Autodesk Inventor part; units mm, degrees
ref_plane "Plano de trabajo3" through (0, 30, 31) normal (0, 0, 1) x (1, 0, 0)
ref_plane "Plano de trabajo4" through (68.3847, 0, 31) normal (1, 0, 0) x (0, 1, 0)
ref_plane "Plano de trabajo5" through (11, 0, 31) normal (0, 0, 1) x (1, 0, 0)
sketch "Boceto1" plane through (0, 0, 0) normal (0, 1, 0) x (-1, 0, 0)
  line L0 (0, 0) -> (-22, 0)
  line L1 (-22, 0) -> (-22, 62)
  line L2 (-22, 62) -> (0, 62)
  line L3 (0, 62) -> (0, 0)
  dimension "d0" = 62
  dimension "d1" = 22
extrude "Extrusión1" add sketch "Boceto1" along normal blind 30
sketch "Boceto2" plane through (22, 0, 62) normal (1, 0, 0) x (0, 0, -1)
  line L0 (62, 0) -> (0, 0)
  line L1 (62, 0) -> (62, 30)
  line L2 (0, 30) -> (62, 30)
  line L3 (0, 0) -> (0, 30)
  line L4 (2, 28) -> (60, 28)
  line L5 (60, 28) -> (60, 2)
  line L6 (60, 2) -> (2, 2)
  line L7 (2, 2) -> (2, 28)
  dimension "d4" = 2
  dimension "d5" = 2
  dimension "d6" = 2
  dimension "d7" = 2
extrude "Extrusión2" cut sketch "Boceto2" against normal blind 30 contours L4 L5 L6 L7
sketch "Boceto3" plane through (0, 0, 0) normal (0, -1, 0) x (1, 0, 0)
  line L0 (0, 0) -> (22, 0)
  line L1 (22, 62) -> (0, 62)
  line L2 (22, 62) -> (7, 62)
  line L3 (7, 62) -> (7, 31)
  circle A0 centre (7, 31) radius 1
  dimension "d10" = 15
  dimension "d11" = 31
  dimension "d12" = 2
extrude "Extrusión3" cut sketch "Boceto3" against normal blind 15
sketch "Boceto4" plane through (0, 0, 62) normal (0, 0, 1) x (1, 0, 0)
  line L0 (22, 0) -> (0, 0)
  line L1 (22, 0) -> (22, 30)
  line L2 (0, 30) -> (22, 30)
  line L3 (0, 0) -> (0, 30)
sketch "Boceto5" plane through (0, 0, 62) normal (0, 0, 1) x (1, 0, 0)
  line L0 (22, 0) -> (0, 0)
  line L1 (22, 0) -> (22, 30)
  line L2 (0, 30) -> (22, 30)
  line L3 (0, 0) -> (0, 30)
sketch "Boceto7" plane through (0, 0, 62) normal (0, 0, 1) x (1, 0, 0)
  line L0 (22, 0) -> (0, 0)
  line L1 (22, 0) -> (22, 30)
  line L2 (0, 30) -> (22, 30)
  line L3 (0, 0) -> (0, 30)
  line L4 (0, 30) -> (22, 30)
  line L5 (22, 30) -> (22, 0)
  line L6 (22, 0) -> (0, 0)
  line L7 (0, 0) -> (0, 30)
  line L8 (22, 0) -> (11, 0)
  line L9 (11, 0) -> (11, 15)
  line L10 (11, 15) -> (22, 15)
  line L11 (22, 15) -> (22, 0)
  dimension "d17" = 15
  dimension "d18" = 11
sketch "Boceto9" plane through (0, 0, 62) normal (0, 0, 1) x (1, 0, 0)
  line L0 (22, 0) -> (0, 0)
  line L1 (22, 0) -> (22, 30)
  line L2 (0, 30) -> (22, 30)
  line L3 (0, 0) -> (0, 30)
sketch "Boceto10" plane through (22, 0, 62) normal (1, 0, 0) x (0, 0, -1)
  line L0 (62, 0) -> (0, 0)
  line L1 (0, 30) -> (62, 30)
  line L2 (0, 30) -> (31, 30) construction
  line L3 (31, 30) -> (31, 0) construction
  line L4 (0, 0) -> (-20, 0)
  line L5 (-20, 0) -> (-20, 15)
  line L6 (-20, 15) -> (0, 15)
  line L7 (0, 15) -> (0, 0)
  line L8 (62, 0) -> (62, 30)
  line L9 (62, 0) -> (82, 0)
  line L10 (82, 0) -> (82, 15)
  line L11 (82, 15) -> (62, 15)
  line L12 (0, 30) -> (62, 30)
  line L13 (62, 30) -> (62, 0)
  line L14 (62, 0) -> (0, 0)
  line L15 (0, 0) -> (0, 30)
  line L16 (2, 28) -> (60, 28)
  line L17 (60, 28) -> (60, 2)
  line L18 (60, 2) -> (2, 2)
  line L19 (2, 2) -> (2, 28)
  dimension "d20" = 31
  dimension "d21" = 20
  dimension "d22" = 15
extrude "Extrusión4" add sketch "Boceto10" against normal blind 11 contours L4 L5 L6 L7
ref_plane "Plano de trabajo3" through (0, 30, 31) normal (0, 0, 1) x (1, 0, 0)
mirror "Simetría1" about plane through (0, 30, 31) normal (0, 0, 1) of "Extrusión4"
sketch "Boceto11" plane through (0, 0, 0) normal (0, -1, 0) x (1, 0, 0)
  line L0 (11, 0) -> (11, -20)
  line L1 (0, 62) -> (0, 0)
  line L2 (11, 82) -> (33, 82)
  line L3 (33, 82) -> (33, 84)
  line L4 (33, 84) -> (11, 84)
  line L5 (11, 84) -> (11, 82)
  line L6 (0, 31) -> (103.8517, 31) construction
  line L7 (11, 62) -> (11, 0) construction
  circle A0 centre (11, 31) radius 57.3847 construction
  line L8 (33, 84) -> (51.3255, 71.8272)
  line L9 (51.3255, 71.8272) -> (68.3847, 31)
  line L10 (33, 82) -> (50.3824, 70.4536)
  line L11 (50.3824, 70.4536) -> (66.8677, 31)
  line L12 (68.3847, 31) -> (66.8677, 31)
  line L13 (11, -20) -> (33, -20)
  line L14 (33, -20) -> (33, -22)
  line L15 (33, -22) -> (11, -22)
  line L16 (11, -22) -> (11, -20)
  line L17 (33, -22) -> (51.3255, -9.8272)
  line L18 (51.3255, -9.8272) -> (68.3847, 31)
  line L19 (33, -20) -> (50.3824, -8.4536)
  line L20 (50.3824, -8.4536) -> (66.8677, 31)
  dimension "d25" = 22
  dimension "d26" = 2
  dimension "d27" = 22
  dimension "d28" = 39.4536
extrude "Extrusión5" add sketch "Boceto11" against normal blind 100
ref_plane "Plano de trabajo4" through (68.3847, 0, 31) normal (1, 0, 0) x (0, 1, 0)
sketch "Boceto12" plane through (68.3847, 0, 31) normal (1, 0, 0) x (0, 1, 0)
  point P0 (0, -31)
sketch "Boceto13" plane through (68.3847, 0, 31) normal (1, 0, 0) x (0, 1, 0)
  line L0 (0, 40.8272) -> (0, 53)
  line L1 (0, 40.8272) -> (100, 40.8272)
  line L2 (100, 53) -> (100, 40.8272)
  line L3 (0, 53) -> (100, 53)
  line L4 (0, 0) -> (0, 40.8272)
  line L5 (0, 0) -> (100, 0)
  line L6 (100, 40.8272) -> (100, 0)
  line L7 (0, 40.8272) -> (100, 40.8272)
  line L8 (0, -40.8272) -> (0, 0)
  line L9 (0, -40.8272) -> (100, -40.8272)
  line L10 (100, 0) -> (100, -40.8272)
  line L11 (0, 0) -> (100, 0)
  line L12 (0, -53) -> (0, -40.8272)
  line L13 (0, -53) -> (100, -53)
  line L14 (100, -40.8272) -> (100, -53)
  line L15 (0, -40.8272) -> (100, -40.8272)
  line L16 (0, 0) -> (20, 0) construction
  line L17 (0, -51) -> (100, -51)
  line L18 (20, 0) -> (32.1544, -40.8272)
  line L19 (32.1544, -40.8272) -> (53.0672, -51)
  line L20 (32.1544, -40.8272) -> (42.1544, -40.8272) construction
  line L21 (20, 0) -> (40, 0) construction
  line L22 (40, 0) -> (42.1544, -40.8272)
  line L23 (42.1544, -40.8272) -> (53.0672, -51)
  line L24 (40, 0) -> (20, 0)
  line L25 (20, 0) -> (0, 0)
  line L26 (42.1544, -40.8272) -> (32.1544, -40.8272)
  line L27 (0, 51) -> (100, 51)
  line L28 (20, 0) -> (32.1544, 40.8272)
  line L29 (32.1544, 40.8272) -> (53.0672, 51)
  line L30 (40, 0) -> (42.1544, 40.8272)
  line L31 (42.1544, 40.8272) -> (53.0672, 51)
  point P0 (0, -31)
  dimension "d32" = 20
  dimension "d33" = 10
  dimension "d34" = 20
  dimension "d35" = 20.9128
extrude "Extrusión6" cut sketch "Boceto13" against normal blind 40 contours L5 L22 L9 L18 | L9 L23 L19
ref_plane "Plano de trabajo5" through (11, 0, 31) normal (0, 0, 1) x (1, 0, 0)
mirror "Simetría2" about plane through (11, 0, 31) normal (0, 0, 1) of "Extrusión6"
sketch "Boceto14" plane through (68.3847, 0, 31) normal (1, 0, 0) x (0, 1, 0)
  line L0 (32.1544, 40.8272) -> (53.0672, 51)
  line L1 (53.0672, 51) -> (42.1544, 40.8272)
  line L2 (42.1544, 40.8272) -> (100, 40.8272)
  line L3 (100, 53) -> (100, 40.8272)
  line L4 (0, 53) -> (100, 53)
  line L5 (0, 40.8272) -> (0, 53)
  line L6 (0, 40.8272) -> (32.1544, 40.8272)
  line L7 (42.1544, 40.8272) -> (40, 0)
  line L8 (40, 0) -> (100, 0)
  line L9 (100, 40.8272) -> (100, 0)
  line L10 (42.1544, 40.8272) -> (100, 40.8272)
  line L11 (40, 0) -> (42.1544, -40.8272)
  line L12 (42.1544, -40.8272) -> (100, -40.8272)
  line L13 (100, 0) -> (100, -40.8272)
  line L14 (40, 0) -> (100, 0)
  line L15 (53.0672, -51) -> (32.1544, -40.8272)
  line L16 (0, -40.8272) -> (32.1544, -40.8272)
  line L17 (0, -53) -> (0, -40.8272)
  line L18 (0, -53) -> (100, -53)
  line L19 (100, -40.8272) -> (100, -53)
  line L20 (42.1544, -40.8272) -> (100, -40.8272)
  line L21 (42.1544, -40.8272) -> (53.0672, -51)
  line L22 (32.1544, -40.8272) -> (20, 0)
  line L23 (0, 0) -> (20, 0)
  line L24 (0, -40.8272) -> (0, 0)
  line L25 (0, -40.8272) -> (32.1544, -40.8272)
  line L26 (20, 0) -> (32.1544, 40.8272)
  line L27 (0, 40.8272) -> (32.1544, 40.8272)
  line L28 (0, 0) -> (0, 40.8272)
  line L29 (0, 0) -> (20, 0)
  line L30 (100, 53) -> (80, 53)
  line L31 (80, 53) -> (80, -53)
  line L32 (100, -53) -> (100, 53)
  line L33 (80, -53) -> (100, -53)
  point P0 (0, -31)
  dimension "d38" = 20
extrude "Extrusión7" cut sketch "Boceto14" against normal blind 40 contours L31 L4 L3 L2 | L2 L9 L8 L31 | L8 L13 L12 L31 | L12 L19 L18 L31
sketch "Boceto15" plane through (0, 30, 0) normal (0, 1, 0) x (1, 0, 0)
  line L0 (0, 0) -> (0, -62)
  line L1 (22, -62) -> (22, 0)
  line L2 (0, -31) -> (22, -31) construction
  line L3 (22, -31) -> (22, -19.5) construction
  line L4 (22, -31) -> (22, -42.5) construction
  line L5 (0, -19.5) -> (55, -19.5)
  line L6 (55, -19.5) -> (55, -14.5)
  line L7 (55, -14.5) -> (22, -14.5)
  line L8 (22, -14.5) -> (22, -9.5)
  line L9 (22, -9.5) -> (0, -9.5)
  line L10 (0, -19.5) -> (0, -9.5)
  line L11 (0, -9.5) -> (0, -19.5)
  line L12 (0, -42.5) -> (55, -42.5)
  line L13 (55, -42.5) -> (55, -47.5)
  line L14 (55, -47.5) -> (22, -47.5)
  line L15 (22, -47.5) -> (22, -52.5)
  line L16 (22, -52.5) -> (0, -52.5)
  line L17 (0, -52.5) -> (0, -42.5)
  dimension "d41" = 11.5
  dimension "d42" = 11.5
  dimension "d43" = 55
  dimension "d44" = 5
  dimension "d45" = 5
extrude "Extrusión8" add sketch "Boceto15" along normal blind 25 contours L9 L1 L5 L0 | L12 L1 L16 L0 | L1 L7 L6 L5 | L12 L13 L14 L1
ref_plane "Plano de trabajo6" through (55, 42.5, 47.5) normal (1, 0, 0) x (0, 0, -1)
sketch "Boceto16" plane through (55, 42.5, 47.5) normal (1, 0, 0) x (0, 0, -1)
  line L0 (28, -12.5) -> (33, -12.5)
  line L1 (33, -12.5) -> (33, 12.5)
  line L2 (28, 12.5) -> (33, 12.5)
  line L3 (28, -12.5) -> (28, 12.5)
  line L4 (0, -12.5) -> (5, -12.5)
  line L5 (5, -12.5) -> (5, 12.5)
  line L6 (0, 12.5) -> (5, 12.5)
  line L7 (0, -12.5) -> (0, 12.5)
  line L8 (0, -12.5) -> (10, -12.5)
  line L9 (10, -12.5) -> (10, 12.5)
  line L10 (10, 12.5) -> (0, 12.5)
  line L11 (0, 12.5) -> (0, -12.5)
  line L12 (5, 0) -> (16.5, 0) construction
  line L13 (-12.5, -40.5) -> (-12.5, -14.5) construction
  line L14 (-12.5, -14.5) -> (45.5, -14.5) construction
  line L15 (45.5, -14.5) -> (45.5, -40.5) construction
  line L16 (45.5, -40.5) -> (-12.5, -40.5) construction
  line L17 (67.5, -42.5) -> (-34.5, -42.5) construction
  line L18 (67.5, -27.5) -> (67.5, -42.5) construction
  line L19 (47.5, -27.5) -> (67.5, -27.5) construction
  line L20 (47.5, -27.5) -> (47.5, -12.5) construction
  line L21 (38, -12.5) -> (47.5, -12.5) construction
  line L22 (38, -12.5) -> (38, 12.5) construction
  line L23 (33, 12.5) -> (38, 12.5) construction
  line L24 (33, -12.5) -> (33, 12.5) construction
  line L25 (28, -12.5) -> (33, -12.5) construction
  line L26 (5, -12.5) -> (28, -12.5) construction
  line L27 (0, -12.5) -> (5, -12.5) construction
  line L28 (0, -12.5) -> (0, 12.5) construction
  line L29 (-5, 12.5) -> (0, 12.5) construction
  line L30 (-5, -12.5) -> (-5, 12.5) construction
  line L31 (-14.5, -12.5) -> (-5, -12.5) construction
  line L32 (-14.5, -27.5) -> (-14.5, -12.5) construction
  line L33 (-14.5, -27.5) -> (-34.5, -27.5) construction
  line L34 (-34.5, -27.5) -> (-34.5, -42.5) construction
  line L35 (16.5, -12.5) -> (16.5, -3.1507) construction
  line L36 (33, -12.5) -> (28, -12.5)
  line L37 (33, 12.5) -> (28, 12.5)
  line L38 (33, -12.5) -> (33, 12.5)
  line L39 (33, -12.5) -> (23, -12.5)
  line L40 (23, -12.5) -> (23, 12.5)
  line L41 (23, 12.5) -> (33, 12.5)
  point P0 (47.5, -42.5)
  dimension "d49" = 25
  dimension "d50" = 11.5
  dimension "d51" = 11.5
extrude "Extrusión9" add sketch "Boceto16" along normal blind 2 contours L7 L6 L5 L4 | L5 L10 L9 L8
ref_plane "Plano de trabajo7" through (33, 0, 31) normal (0, 0, -1) x (-1, 0, 0)
mirror "Simetría3" about plane through (33, 0, 31) normal (0, 0, -1) of "Extrusión9"
ref_plane "Plano de trabajo8" through (55, 42.5, 24.5) normal (-1, 0, 0) x (0, 0, 1)
sketch "Boceto17" plane through (55, 42.5, 24.5) normal (-1, 0, 0) x (0, 0, 1)
  line L0 (-5, -12.5) -> (-5, 12.5)
  line L1 (-5, -12.5) -> (0, -12.5)
  line L2 (0, -12.5) -> (0, 12.5)
  line L3 (0, 12.5) -> (-5, 12.5)
  line L4 (18, -12.5) -> (18, 12.5)
  line L5 (13, 12.5) -> (18, 12.5)
  line L6 (13, -12.5) -> (13, 12.5)
  line L7 (18, -12.5) -> (13, -12.5)
  line L8 (18, -12.5) -> (18, -5.5) construction
  line L9 (18, -5.5) -> (15.5, -5.5) construction
  circle A0 centre (15.5, -5.5) radius 1.5 construction
  circle A1 centre (15.5, -5.5) radius 1.5
  circle A2 centre (15.5, 6.5997) radius 1.5
  circle A3 centre (-2.5, 6.5997) radius 1.5
  circle A4 centre (-2.5, -5.5) radius 1.5
  point P0 (-24.5, -42.5)
  dimension "d54" = 7
  dimension "d55" = 2.5
  dimension "d56" = 3
  dimension "d57" = 3
  dimension "d58" = 3
  dimension "d59" = 3
  dimension "d60" = 3
extrude "Extrusión10" cut sketch "Boceto17" against normal blind 5 contours A1 | A2 | A3 | A4
sketch "Boceto18" plane through (0, 0, 0) normal (0, -1, 0) x (1, 0, 0)
  line L0 (0, 62) -> (-88, 62)
  line L1 (-88, 62) -> (-88, 53.488)
  line L2 (-88, 53.488) -> (0, 53.488)
  line L3 (0, 53.488) -> (0, 62)
  dimension "d63" = 88
extrude "Extrusión11" add sketch "Boceto18" against normal blind 2
mirror "Simetría4" about plane through (33, 0, 31) normal (0, 0, -1) of "Extrusión11"
fillet "Empalme1" radius 2 1 edges at (27.5, 55, 19.5)
fillet "Empalme2" radius 2 1 edges at (27.5, 55, 42.5)
fillet "Empalme3" radius 2 1 edges at (56, 55, 37.5)
fillet "Empalme4" radius 2 1 edges at (56, 55, 24.5)
fillet "Empalme5" radius 2 1 edges at (11, 15, 72)
fillet "Empalme6" radius 2 1 edges at (11, 15, -10)
fillet "Empalme7" radius 2 1 edges at (22, 15, 72)
fillet "Empalme8" radius 2 1 edges at (22, 15, -10)
properties part number "Face" material "Madera (cerezo)"
Read the model definition and answer for the solid it produces. Units are mm, in the model's axes. A direction names the side the tool comes from. Round coordinates to 2 decimals unless told otherwise and drop trailing zeros. Order: outer loops, then holes, each group sorted by start corner. A loop starts at its lowest first (then second) coordinate and runs counter-clockwise, first axis right, second up. Notation, with made-up numbers: (89, 77.25) - (99, 77.25) arc R20 ccw to (99, 89.25) - close; hole circle Ø4 at (86, 23.5). An arc over 180 degrees is marked (long way). Use one line per item in the form item = value. Start each with the question number.
(1) The part is cut by section C-C (y = 63.5). Give the vertices of the cut face in (x, z).
(2) The part is cut by section D-D (x = 17.5). Give the vertices of the cut face in (y, z).
(3) The part is cut by section A-A (y = 87). Give the vertices of the cut face in (x, z).
(4) Flat-ended cylindrical pins translate along their axes: pin 1 Ø18.5 at (x, z) = (-8, 23) entering from +Y; pin 2 Ø3 at (y, z) = (80, -6.5) entering from -X; pin 3 Ø1.5 at (y, z) = (54, 26) entering from +X. Find the tip coordinate at first contact, or state that the pin passes through.
(5) For faces 1 (the face through (11, 42, 9.5)), 2 (the face through (11, 28, 83)), 3 (the face through (64.8, 80, 39.1)), determine the directions among +Z, -Z, +X, -X, +Y, -Y from which every point of the face is accessible in a straight line to the end or side of a thin tool.
(6) Find the intervals of material crossed by line 1 along Y through (x, z) = (56, 40); line 2 along Y through (x, z) = (2, 57); line 3 along Z through (x, y) = (11.5, 55.5), in increasing order. Write a range as from..to.
(7) Determine the mould class of faces 4 (the face through (22, 49, -22)), 5 (the face through (22, 49, 84)), 6 (the face through (0, 28.4, 31.1)), 7 (the face through (39, 30, 45)) for opening direction Z: +Z half, -Z half, draft (parallel to the pull), parting line (faces both ways), or undercut.
(8) The part is cut by section B-B (x = -33). Give the vertices of the cut face in (y, z), then the cut area to 3 significant figures.
Checked values:
q1.outline = (11, -22) - (33, -22) - (51.33, -9.83) - (68.38, 31) - (51.33, 71.83) - (33, 84) - (11, 84) - (11, 82) - (33, 82) - (50.38, 70.45) - (66.87, 31) - (50.38, -8.45) - (33, -20) - (11, -20) - close
q2.outline = (0, -22) - (100, -22) - (100, -20) - (15, -20) - (15, 0) - (30, 0) - (30, 9.5) - (55, 9.5) - (55, 17.5) arc R2 ccw to (53, 19.5) - (30, 19.5) - (30, 42.5) - (53, 42.5) arc R2 ccw to (55, 44.5) - (55, 52.5) - (30, 52.5) - (30, 62) - (15, 62) - (15, 82) - (100, 82) - (100, 84) - (0, 84) - close; hole (2, 2) - (28, 2) - (28, 60) - (2, 60) - close
q3.outline = (11, -22) - (28.38, -22) - (28.38, -20) - (11, -20) - close; (11, 82) - (28.38, 82) - (28.38, 84) - (11, 84) - close
q4.pin_1 = 54.81
q4.pin_2 = 50.57
q4.pin_3 = 66.61
q5.face_1 = -X, +Y
q5.face_2 = +Z, -X, +Y, -Y
q5.face_3 = +Z, -Z, +X, +Y
q6.line_1 = 30..35.5, 38.5..47.6, 50.6..55
q6.line_2 = 0..2, 28..30
q6.line_3 = -22..-20, 82..84
q7.face_4 = -Z half
q7.face_5 = +Z half
q7.face_6 = draft
q7.face_7 = undercut
q8.outline = (0, 0) - (2, 0) - (2, 8.51) - (0, 8.51) - close; (0, 53.49) - (2, 53.49) - (2, 62) - (0, 62) - close
q8.area = 34.0 mm^2
